```python
from build123d import *

# Parameters (mm, degrees)
BOSS_EXTRUDE1_DEPTH      = 2
BOSS_EXTRUDE1_DEPTH_BACK = 3
SKETCH1_R                = 16
SKETCH1_R_2              = 1
SKETCH2_R                = 4.85
SKETCH2_R_2              = 2.85
BOSS_EXTRUDE3_DEPTH      = 3
SKETCH5_R                = 2
CUT_EXTRUDE2_DEPTH       = 1


with BuildPart() as part:
    # Sketch1 → Boss-Extrude1 (new, two sides: drawn at the far end of the back side and taken through both)
    with BuildSketch(Plane(origin=(0, 0, 0), x_dir=(1, 0, 0), z_dir=(0, 1, 0)).offset(-BOSS_EXTRUDE1_DEPTH_BACK)):
        with Locations(Location((0, 0, 0), (0, 0, 270))):
            Circle(SKETCH1_R)
        with Locations(Location((0, 0, 0), (0, 0, 270))):
            Circle(SKETCH1_R_2, mode=Mode.SUBTRACT)
        with Locations(Location((-13.5, 0, 0), (0, 0, 270))):
            Circle(SKETCH1_R_2, mode=Mode.SUBTRACT)
        with Locations(Location((-4.171729424, 12.83926297, 0), (0, 0, 270))):
            Circle(SKETCH1_R_2, mode=Mode.SUBTRACT)
        with Locations(Location((10.921729424, 7.935100906, 0), (0, 0, 270))):
            Circle(SKETCH1_R_2, mode=Mode.SUBTRACT)
        with Locations(Location((10.921729424, -7.935100906, 0), (0, 0, 270))):
            Circle(SKETCH1_R_2, mode=Mode.SUBTRACT)
        with Locations(Location((-4.171729424, -12.83926297, 0), (0, 0, 270))):
            Circle(SKETCH1_R_2, mode=Mode.SUBTRACT)
    extrude(amount=BOSS_EXTRUDE1_DEPTH + BOSS_EXTRUDE1_DEPTH_BACK)

    # Sketch2 → Boss-Extrude3 (add)
    with BuildSketch(Plane(origin=(0, 2, 0), x_dir=(1, 0, 0), z_dir=(0, 1, 0))):
        with Locations(Location((0, 0, 0), (0, 0, 270))):
            Circle(SKETCH2_R)
        with Locations(Location((0, 0, 0), (0, 0, 270))):
            Circle(SKETCH2_R_2, mode=Mode.SUBTRACT)
    extrude(amount=BOSS_EXTRUDE3_DEPTH)

    # Sketch5 → Cut-Extrude2 (cut)
    with BuildSketch(Plane.XZ.offset(3)):
        with Locations(Location((0, 0, 0), (0, 0, 270))):
            Circle(SKETCH5_R)
    extrude(amount=-CUT_EXTRUDE2_DEPTH, mode=Mode.SUBTRACT)


solid = part.part
```
Design review of the part built by this model. Coordinates are the model's own, in mm. A direction names the side the tool comes from. Give positions to 0.01 mm unless a question says otherwise; leave off trailing zeros. Write each loop counter-clockwise with the first axis right and the second up, starting at its lowest first coordinate (ties: lowest second). Pieces come first, ordered by that corner, then holes. Notation, with made-up numbers: (64, 82.5) - (96, 82.5) arc R31 ccw to (96, 120.5) - close; hole circle Ø2 at (47, 37.5). An arc over 180 degrees is marked (long way). Return JSON: item names as keys, results as strings. Group by question number.
(1) To check wall thickness, follow probe 1 along X at (y, z) = (-0.2, 0); probe 2 along Z at (x, y) = (-0.5, 0.5); probe 3 along Y at (x, z) = (7, 9). State the ranges of each line that lie inside material, in increasing order.
(2) We need section C-C, the plane y = -1.5. Give the boundary of the cut face in (x, z).
(3) We need section D-D, the plane z = 12.5. Give the boundary of the cut face in (x, y), then the cut area to 3 significant figures.
(4) We need section B-B, the plane z = 0. Give the boundary of the cut face in (x, y), then the cut area to 3 significant figures.
(5) Insertion check: pin 1 (3 mm diameter, centred on x = -4.17, z = -12.84, fed in from +Y); pin 2 (1 mm diameter, centred on x = 6.5, y = -2, fed in from +Z); pin 3 (1.2 mm diameter, centred on x = 1, z = -0.5, fed in from -Y). Each pin has a flat end and moves straight along its axis. Give the tip position at first contact, or say it passes through.
(6) Mouldability with a two-part tool opening along X and no side actions: class faces 1 (the flat face through (0, -3, 3)), 2 (the cylindrical face through (10.966, -0.535, 6.936)), 3 (the cylindrical face through (1.457, 3.479, 4.626)) as +X half, -X half, draft (parallel to the pull), parting line (faces both ways), or undercut.
(7) Machinability: for faces 4 (the cylindrical face through (-1.734, 3.479, -2.262)), 5 (the cylindrical face through (-1.952, -2.507, 0.434)), 6 (the flat face through (-3.2, 5, -0.1)), which of the approach directions +Z, -Z, +X, -X, +Y, -Y give a long, thin tool a straight path to every point of the face, cutting with its end or side? Answer none if there is none.
(8) We need section A-A, the plane x = 0. Give the boundary of the cut face in (y, z), then the cut area to 3 significant figures.
Reported:
{
 "1": {"probe 1": "x = -16 to -14.5, -12.5 to -1, 1 to 16", "probe 2": "z = -15.99 to -0.87, 0.87 to 15.99", "probe 3": "y = -3 to 2"},
 "2": {"outline": "circle Ø32 at (0, 0); hole circle Ø2 at (-13.5, 0); hole circle Ø2 at (-4.17, -12.84); hole circle Ø2 at (-4.17, 12.84); hole circle Ø2 at (0, 0); hole circle Ø2 at (10.92, -7.94); hole circle Ø2 at (10.92, 7.94)"},
 "3": {"outline": "(-9.99, -3) - (-5.11, -3) - (-5.11, 2) - (-9.99, 2) - close; (-3.23, -3) - (9.99, -3) - (9.99, 2) - (-3.23, 2) - close", "area": "90.5 mm2"},
 "4": {"outline": "(-16, -3) - (-14.5, -3) - (-14.5, 2) - (-16, 2) - close; (-12.5, -3) - (-2, -3) - (-2, -2) - (-1, -2) - (-1, 2) - (-2.85, 2) - (-2.85, 5) - (-4.85, 5) - (-4.85, 2) - (-12.5, 2) - close; (1, -2) - (2, -2) - (2, -3) - (16, -3) - (16, 2) - (4.85, 2) - (4.85, 5) - (2.85, 5) - (2.85, 2) - (1, 2) - close", "area": "150 mm2"},
 "5": {"pin 1": "stops at y = 2", "pin 2": "stops at z = 14.83", "pin 3": "stops at y = -2"},
 "6": {"face 1": "draft", "face 2": "undercut", "face 3": "parting line"},
 "7": {"face 4": "+Y", "face 5": "-Y", "face 6": "+Z, -Z, +X, -X, +Y"},
 "8": {"outline": "(-3, -16) - (2, -16) - (2, -4.85) - (5, -4.85) - (5, -2.85) - (2, -2.85) - (2, -1) - (-2, -1) - (-2, -2) - (-3, -2) - close; (-3, 2) - (-2, 2) - (-2, 1) - (2, 1) - (2, 2.85) - (5, 2.85) - (5, 4.85) - (2, 4.85) - (2, 16) - (-3, 16) - close", "area": "160 mm2"}
}
